Autodesk Inventor part; units mm, degrees
ref_plane "YZ Plane" through (0, 0, 0) normal (1, 0, 0) x (0, 1, 0)
ref_plane "XZ Plane" through (0, 0, 0) normal (0, 1, 0) x (-1, 0, 0)
ref_plane "XY Plane" through (0, 0, 0) normal (0, 0, 1) x (1, 0, 0)
sketch "Sketch1" plane through (0, 0, 0) normal (0, 1, 0) x (-1, 0, 0)
  line L0 (0, 0) -> (-304.8, 0)
  line L1 (-304.8, 0) -> (-304.8, -228.6)
  line L2 (-304.8, -228.6) -> (0, -228.6)
  line L3 (0, -228.6) -> (0, 0)
  line L4 (-12.7, -12.7) -> (-292.1, -12.7) construction
  line L5 (-292.1, -12.7) -> (-292.1, -215.9) construction
  line L6 (-292.1, -215.9) -> (-12.7, -215.9) construction
  line L7 (-12.7, -215.9) -> (-12.7, -12.7) construction
  circle A0 centre (-12.7, -12.7) radius 2.0701
  circle A1 centre (-12.7, -215.9) radius 2.0701
  circle A2 centre (-292.1, -12.7) radius 2.0701
  circle A3 centre (-292.1, -215.9) radius 2.0701
  circle A4 centre (-114.3, -12.7) radius 2.0701
  circle A5 centre (-63.5, -12.7) radius 2.0701
  circle A6 centre (-241.3, -12.7) radius 2.0701
  circle A7 centre (-12.7, -63.5) radius 2.0701
  circle A8 centre (-12.7, -114.3) radius 2.0701
  circle A9 centre (-12.7, -165.1) radius 2.0701
  circle A10 centre (-190.5, -215.9) radius 2.0701
  circle A11 centre (-63.5, -215.9) radius 2.0701
  circle A12 centre (-114.3, -215.9) radius 2.0701
  circle A13 centre (-292.1, -63.5) radius 2.0701
  circle A14 centre (-292.1, -114.3) radius 2.0701
  circle A15 centre (-292.1, -165.1) radius 2.0701
  circle A16 centre (-190.5, -12.7) radius 2.0701
  circle A17 centre (-241.3, -215.9) radius 2.0701
  point P0 (-12.7, -114.3)
  dimension "d0" = 304.8
  dimension "d1" = 228.6
  dimension "d2" = 12.7
  dimension "d3" = 12.7
  dimension "d4" = 12.7
  dimension "d5" = 12.7
  dimension "d6" = 4.1402
  dimension "d8" = 50.8
  dimension "d9" = 50.8
  dimension "d10" = 50.8
  dimension "d11" = 50.8
  dimension "d12" = 50.8
  dimension "d13" = 101.6
  dimension "d14" = 101.6
extrude "Extrusion1" add sketch "Sketch1" along normal blind 1.6002
sketch "Sketch2" plane through (0, 1.6002, 0) normal (0, 1, 0) x (1, 0, 0)
  line L0 (57.15, 88.9) -> (57.15, 50.8) construction
  line L1 (54.7687, 88.9) -> (54.7687, 50.8)
  line L2 (59.5312, 50.8) -> (59.5312, 88.9)
  arc A0 (59.5312, 88.9) -> (54.7687, 88.9) centre (57.15, 88.9) ccw
  arc A1 (54.7687, 50.8) -> (59.5312, 50.8) centre (57.15, 50.8) ccw
  line L3 (0, 228.6) -> (0, 0)
  line L4 (304.8, 228.6) -> (0, 228.6)
  line L5 (57.15, 177.8) -> (57.15, 139.7) construction
  line L6 (54.7687, 177.8) -> (54.7687, 139.7)
  line L7 (59.5312, 139.7) -> (59.5312, 177.8)
  arc A2 (59.5312, 177.8) -> (54.7687, 177.8) centre (57.15, 177.8) ccw
  arc A3 (54.7687, 139.7) -> (59.5312, 139.7) centre (57.15, 139.7) ccw
  line L8 (252.4125, 177.8) -> (252.4125, 139.7) construction
  line L9 (250.0313, 177.8) -> (250.0313, 139.7)
  line L10 (254.7938, 139.7) -> (254.7938, 177.8)
  arc A4 (254.7938, 177.8) -> (250.0313, 177.8) centre (252.4125, 177.8) ccw
  arc A5 (250.0313, 139.7) -> (254.7938, 139.7) centre (252.4125, 139.7) ccw
  line L11 (252.4125, 88.9) -> (252.4125, 50.8) construction
  line L12 (250.0312, 88.9) -> (250.0312, 50.8)
  line L13 (254.7938, 50.8) -> (254.7938, 88.9)
  arc A6 (254.7938, 88.9) -> (250.0312, 88.9) centre (252.4125, 88.9) ccw
  arc A7 (250.0312, 50.8) -> (254.7938, 50.8) centre (252.4125, 50.8) ccw
  circle A8 centre (34.29, 114.3) radius 2.54
  circle A9 centre (270.51, 114.3) radius 2.54
  line L14 (304.8, 0) -> (304.8, 228.6)
  point P0 (57.15, 69.85)
  point P1 (0, 114.3)
  point P2 (152.4, 228.6)
  point P3 (0, 114.3)
  point P4 (57.15, 158.75)
  point P5 (252.4125, 158.75)
  point P6 (252.4125, 69.85)
  point P7 (250.0313, 158.75)
  point P8 (304.8, 114.3)
  dimension "d17" = 4.7625
  dimension "d18" = 38.1
  dimension "d19" = 25.4
  dimension "d20" = 50.8
  dimension "d21" = 190.5
  dimension "d22" = 95.25
  dimension "d25" = 5.08
  dimension "d26" = 34.29
  dimension "d27" = 34.29
extrude "Extrusion2" cut sketch "Sketch2" against normal blind 25.4
equation "\"d3\" = d2"
equation "\"d4\" = d2"
equation "\"d5\" = d2"
equation "\"d8\" = d9"
equation "\"d14\" = d13"
equation "\"d27\" = d26"
properties part number "BatteryPlate" material "Stainless Steel"
Read the model definition and answer for the solid it produces. Units are mm, in the model's axes. Coordinates: 2 decimals unless noted, no trailing zeros. Loops run counter-clockwise (first coordinate to the right, second up) from the corner with the lowest first, then second, coordinate; pieces in that order, holes last. Notation, with made-up numbers: (-14, 2.5) -> (33, 2.5) arc R20 cw to (33, 17.5) -> close; hole circle Ø1 at (-34.75, 47.5). An arc over 180 degrees is marked (long way). Write item = value, one per line. Start each with the question number.
1) The part is cut by section A-A, the plane z = -152.5. Determine the outline of the cut face in (x, y), plus the area to 4 significant figures.
2) Find the intervals of material crossed by L1, parallel to Z at x = 114.3, y = 0.8; L2, parallel to Z at x = 292.1, y = 0.7; L3, parallel to Z at x = 34.29, y = 0.45, in increasing order. Write a range as from..to.
3) The part is cut by section B-B, the plane y = 0.85. State how many separate pieces and enclosed holes the cut face has, plus the area to 3 significant figures.
Result:
q1.outline = (0, 0) -> (54.77, 0) -> (54.77, 1.6) -> (0, 1.6) -> close; (59.53, 0) -> (250.03, 0) -> (250.03, 1.6) -> (59.53, 1.6) -> close; (254.79, 0) -> (304.8, 0) -> (304.8, 1.6) -> (254.79, 1.6) -> close
q1.area = 472.5 mm²
q2.L1 = -228.6..-217.97, -213.83..-14.77, -10.63..0
q2.L2 = -228.6..-217.97, -213.83..-167.17, -163.03..-116.37, -112.23..-65.57, -61.43..-14.77, -10.63..0
q2.L3 = -228.6..-116.84, -111.76..0
q3.separate_pieces = 1
q3.enclosed_holes = 24
q3.area = 68,600 mm²
